Can you work these out from the drawing? Everything is in mm from the part's minimum corner. Give positions to 0.01 mm unless a question says otherwise; leave off trailing zeros. Order: outer loops, then holes, each group sorted by start corner. A loop starts at its lowest first (then second) coordinate and runs counter-clockwise, first axis right, second up. Notation, with made-up numbers: M -38.75,74.25 L -1.75,74.25 A29 cw -1.75,98.25 Z; hole C 2,75.5 d2. An arc over 180 degrees is marked long. Answer as a JSON object with one key per item and string values.
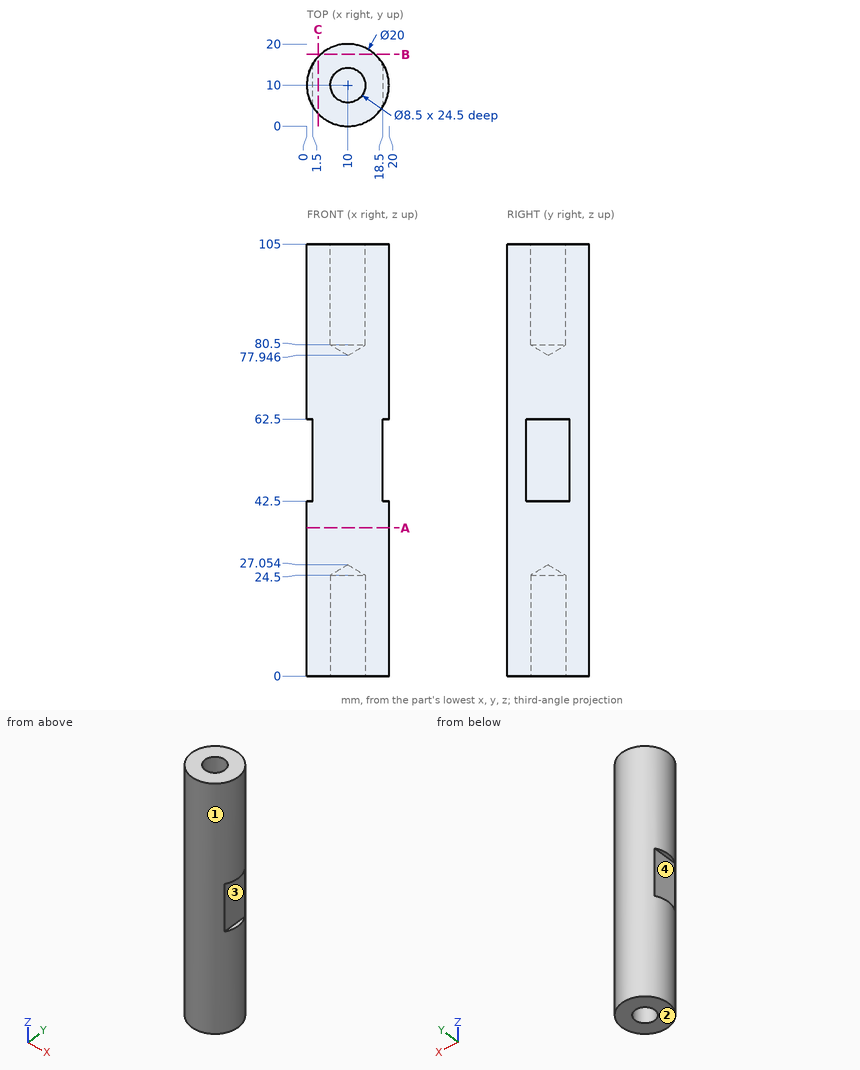
1) I want a section at C-C on x = 2.75. Write out the boundary of the cut face in (y, z).
Results found:
{"outline": "M 3.11,0 L 16.89,0 L 16.89,105 L 3.11,105 Z"}
2) I need wall thicknesses on L1, parallel to Y at x = 10, z = 91; L2, parallel to Z at x = 19.25, y = 10. Which ranges of each line are inside material? Lowest first, please.
Results found:
{"L1": "y = 0 to 5.75, 14.25 to 20", "L2": "z = 0 to 42.5, 62.5 to 105"}
3) I want a section at B-B on y = 17.5. Write out the boundary of the cut face in (x, z) (1 decimal).
Results found:
{"outline": "M 3.4,0 L 16.6,0 L 16.6,105 L 3.4,105 Z"}
4) Thinking about a two-plate mould opening in Z: for the marked faces 1, 2, 3 and 4, which applies, pulls with the +Z half, pulls with the -Z half, needs draft (parallel to the pull), parting line crosses it, or undercut?
Results found:
{"face 1": "needs draft", "face 2": "pulls with the -Z half", "face 3": "undercut", "face 4": "undercut"}
5) I want a section at A-A on z = 36. Write out the boundary of the cut face in (x, y), and give its area (3 significant figures).
Results found:
{"outline": "C 10,10 d20", "area": "314 mm²"}
6) I'm going to push flat-ended pins straight in: pin 1 Ø4 at (x, z) = (16.5, 59) entering from -Y; pin 2 Ø7.5 at (x, y) = (10, 10) entering from -Z; pin 3 Ø1 at (y, z) = (4, 79.5) entering from -X. Where does each tip first touch, or does it pass through?
Results found:
{"pin 1": "stops at y = 1.07", "pin 2": "stops at z = 24.8", "pin 3": "stops at x = 1.65"}
